Work out the finished part from the listing and answer in its coordinate system (mm). Face numbers are marked on the shaded views. Coordinates: 2 decimals unless noted, no trailing zeros. Write each loop counter-clockwise with the first axis right and the second up, starting at its lowest first coordinate (ties: lowest second). Pieces come first, ordered by that corner, then holes. Notation, with made-up numbers: (-17.75, 43.5) - (5.25, 43.5) arc R25 cw to (5.25, 80.5) - close; hole circle Ø9 at (52, -7). An arc over 180 degrees is marked (long way). Answer as a JSON object with one key per item and string values. Group by question number.
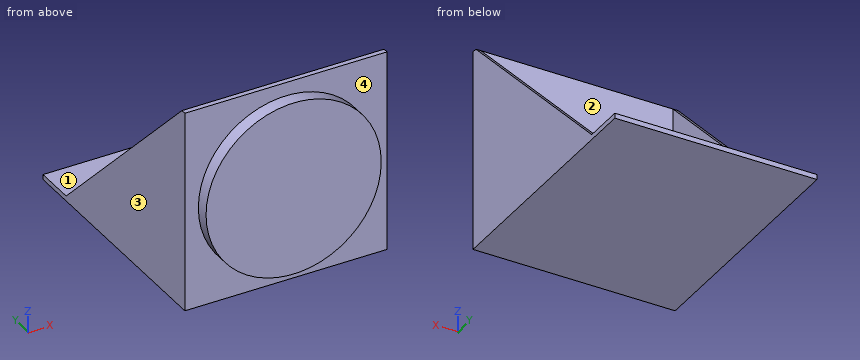
from build123d import *

# Parameters (mm, degrees)
F0_W     = 762
F0_H     = 762
F1_DEPTH = 19.05
F2_W     = 762
F2_H     = 914.4
F3_DEPTH = 19.05
F5_DEPTH = 19.05
F7_DEPTH = 19.05
F8_R     = 330.2
F9_DEPTH = 50.8


with BuildPart() as f1:
    # F0 (on Front) → F1 (new body)
    with BuildSketch(Plane.XZ):
        Rectangle(F0_W, F0_H)
    extrude(amount=F1_DEPTH)

    # F2 (on face) → F3 (join)
    with BuildSketch(Plane(origin=(0, 0, -381), x_dir=(1, 0, 0), z_dir=(0, 0, -1))):
        with Locations((0, -457.2)):
            Rectangle(F2_W, F2_H)
    extrude(amount=-F3_DEPTH)

    # F4 (on face) → F5 (join)
    with BuildSketch(Plane(origin=(-381, 0, 0), x_dir=(0, -1, 0), z_dir=(-1, 0, 0))):
        Polygon((0, 273.05), (0, 381), (-762, -361.95), (-635, -361.95), (0, 257.175), align=None)
        Polygon((0, -361.95), (0, 257.175), (-635, -361.95), align=None)
    extrude(amount=-F5_DEPTH)

    # F6 (on face) → F7 (join)
    with BuildSketch(Plane.YZ.offset(381)):
        Polygon((0, 381), (0, -361.95), (762, -361.95), align=None)
    extrude(amount=-F7_DEPTH)

    # F8 (on face) → F9 (join)
    with BuildSketch(Plane.XZ.offset(19.05)):
        Circle(F8_R)
    extrude(amount=F9_DEPTH)


solid = f1.part
Q1. Flat-ended cylindrical pins translate along their axes: pin 1 Ø1 at (x, y) = (198.5, 239) entering from +Z; pin 2 Ø12 at (x, z) = (217, 22) entering from +Y. Find the tip coordinate at first contact, or state that the pin passes through.
Q2. Section A-A on x = 0 is taken. Determine the outline of the cut face in (y, z), plus the area to 3 significant figures.
Q3. Consider L1, parallel to X at y = 290, z = -332; L2, parallel to Z at x = -218.5, y = 530.5; L3, parallel to Y at x = -162, z = -2. Determine where each line is inside the solid, lowest interval first. Write a range as from..to.
Q4. Section B-B on z = 106.5 is taken. Determine the outline of the cut face in (x, y).
Q5. For a pull along X with two mould halves and no side action, classify the marked faces 1, 2, 3 and 4 as +X half, -X half, draft (parallel to the pull), parting line (faces both ways), or undercut.
Q6. Section C-C on z = -182 is taken. Determine the outline of the cut face in (x, y), plus the area to 3 significant figures.
Q7. Section D-D on x = -287 is taken. Determine the outline of the cut face in (y, z), plus the area to 3 significant figures.
Numbers:
{
 "1": {"pin 1": "stops at z = -361.95", "pin 2": "stops at y = 0"},
 "2": {"outline": "(-69.85, -330.2) - (-19.05, -330.2) - (-19.05, -381) - (914.4, -381) - (914.4, -361.95) - (0, -361.95) - (0, 381) - (-19.05, 381) - (-19.05, 330.2) - (-69.85, 330.2) - close", "area": "65,500 mm²"},
 "3": {"L1": "x = -381..-361.95, 361.95..381", "L2": "z = -381..-361.95", "L3": "y = -69.85..0"},
 "4": {"outline": "(-381, -19.05) - (-312.55, -19.05) - (-312.55, -69.85) - (312.55, -69.85) - (312.55, -19.05) - (381, -19.05) - (381, 281.54) - (361.95, 281.54) - (361.95, 0) - (-361.95, 0) - (-361.95, 281.54) - (-381, 281.54) - close"},
 "5": {"face 1": "undercut", "face 2": "undercut", "face 3": "-X half", "face 4": "draft"},
 "6": {"outline": "(-381, -19.05) - (-275.51, -19.05) - (-275.51, -69.85) - (275.51, -69.85) - (275.51, -19.05) - (381, -19.05) - (381, 577.44) - (361.95, 577.44) - (361.95, 0) - (-361.95, 0) - (-361.95, 577.44) - (-381, 577.44) - close", "area": "64,500 mm²"},
 "7": {"outline": "(-69.85, -163.29) - (-19.05, -163.29) - (-19.05, -381) - (914.4, -381) - (914.4, -361.95) - (0, -361.95) - (0, 381) - (-19.05, 381) - (-19.05, 163.29) - (-69.85, 163.29) - close", "area": "48,500 mm²"}
}
